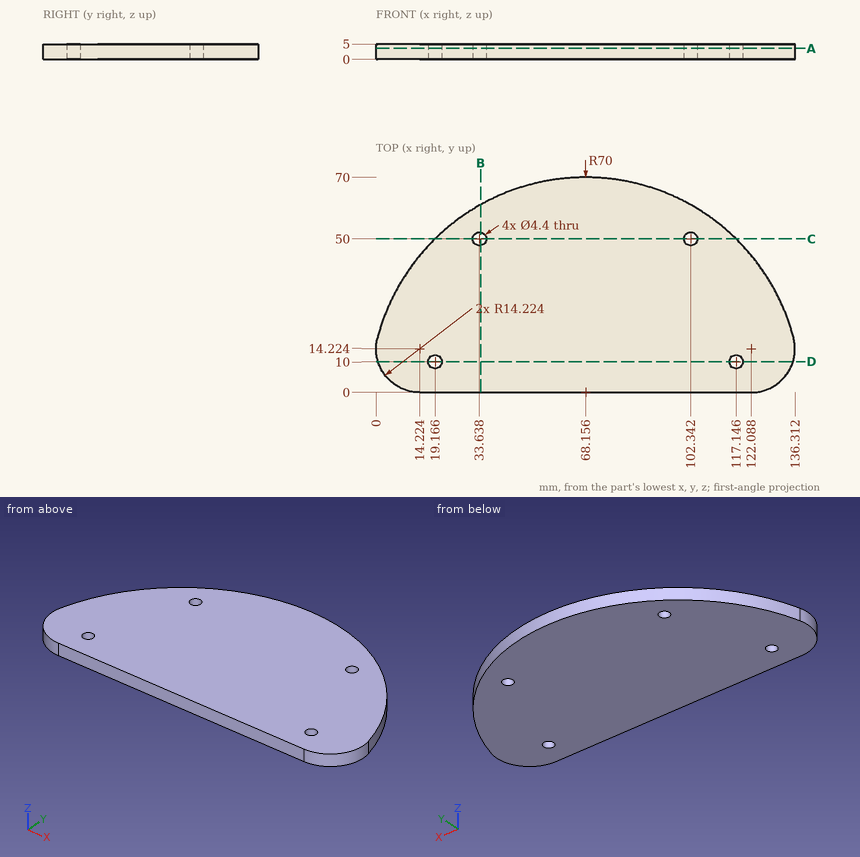
The drawing under review shows one solid part. Ordinate dimensions are in mm from its lowest x, y, z. Give positions to 0.01 mm unless a question says otherwise; leave off trailing zeros. Order: outer loops, then holes, each group sorted by start corner. A loop starts at its lowest first (then second) coordinate and runs counter-clockwise, first axis right, second up. Notation, with made-up numbers: (56.5, 81.5) - (111.5, 81.5) arc R20 ccw to (111.5, 106.5) - close; hole circle Ø6 at (-13, 34). An arc over 180 degrees is marked (long way). Answer as a JSON object with one key per item and string values. Group by question number.
Item 1: Take a section at B-B on x = 34. Give the boundary of the cut face in (y, z), and give its area (3 significant figures).
Item 2: Take a section at A-A on z = 3.55. Give the boundary of the cut face in (x, y) (1 decimal), and give its area (3 significant figures).
Item 3: Take a section at C-C on y = 50. Give the boundary of the cut face in (x, z) (1 decimal), and give its area (3 significant figures).
Item 4: Take a section at D-D on y = 10. Give the boundary of the cut face in (x, z) (1 decimal).
Item 5: Wall thickness on line 1 along X through (y, z) = (51, 2.7) (1 decimal); line 2 along Y through (x, z) = (21, 3.8) (1 decimal); line 3 along Y through (x, z) = (118.5, 1.8) (1 decimal): over which ranges is each line inside the solid? List them lowest first.
Item 6: Clearance check with a flat-ended pin moving along its axis: pin 1 Ø3 at (x, z) = (52, 1) entering from -Y. State where the tip first meets the part, or that it passes through.
Reported:
{
 "1": {"outline": "(0, 0) - (47.83, 0) - (47.83, 5) - (0, 5) - close; (52.17, 0) - (61.1, 0) - (61.1, 5) - (52.17, 5) - close", "area": "284 mm^2"},
 "2": {"outline": "(0.5, 17.9) arc R14.2 ccw to (14.2, 0) - (122.1, 0) arc R14.2 ccw to (135.8, 17.9) arc R70 ccw to start; hole circle Ø4.4 at (19.2, 10); hole circle Ø4.4 at (33.6, 50); hole circle Ø4.4 at (102.3, 50); hole circle Ø4.4 at (117.1, 10)", "area": "7,510 mm^2"},
 "3": {"outline": "(19.2, 0) - (31.4, 0) - (31.4, 5) - (19.2, 5) - close; (35.8, 0) - (100.1, 0) - (100.1, 5) - (35.8, 5) - close; (104.5, 0) - (117.1, 0) - (117.1, 5) - (104.5, 5) - close", "area": "446 mm^2"},
 "4": {"outline": "(0.6, 0) - (17, 0) - (17, 5) - (0.6, 5) - close; (21.4, 0) - (114.9, 0) - (114.9, 5) - (21.4, 5) - close; (119.3, 0) - (135.7, 0) - (135.7, 5) - (119.3, 5) - close"},
 "5": {"line 1": "20.2 to 31.7, 35.6 to 100.4, 104.3 to 116.1", "line 2": "0 to 8.8, 11.2 to 51.7", "line 3": "0 to 8.3, 11.7 to 48.6"},
 "6": {"pin 1": "y = 0"}
}
